from build123d import *

# Parameters (mm, degrees)
F0_R        = 30
F0_R_2      = 5
F1_DEPTH    = 4
F2_R        = 30
F3_R        = 30
F4_T1_DEPTH = 8
F5_R        = 30
F5_R_2      = 24
F6_DEPTH    = 30
F0_R_3      = 13
F7_DEPTH    = 20


# Not quite as in the source:
# - a fillet or chamfer that OpenCascade refuses, or shapes differently, is made with other operations: its cross-section is extruded or revolved along the edge and cut away or added


with BuildPart() as f1:
    # F0 (on Front) → F1 (new body, symmetric)
    with BuildSketch(Plane.XZ):
        with BuildLine():
            ThreePointArc((34.9249194702, -19.5), (38.7104428986, -10.074800772), (40, 0))
            ThreePointArc((40, 0), (38.7104428986, 10.074800772), (34.9249194702, 19.5))
            ThreePointArc((34.9249194702, 19.5), (28.892590505, 27.6625778609), (21, 34.0440890611))
            ThreePointArc((21, 34.0440890611), (0, 40), (-21, 34.0440890611))
            ThreePointArc((-21, 34.0440890611), (-27.6625778609, -28.892590505), (34.9249194702, -19.5))
        make_face()
        Circle(F0_R, mode=Mode.SUBTRACT)
        with BuildLine():
            ThreePointArc((34.9249194702, 19.5), (38.7104428986, 10.074800772), (40, 0))
            ThreePointArc((40, 0), (38.7104428986, -10.074800772), (34.9249194702, -19.5))
            Line((34.9249194702, -19.5), (206.3684774144, -12.4895628079))
            ThreePointArc((206.3684774144, -12.4895628079), (193.3577711699, 0), (206.3684774144, 12.4895628079))
            Line((206.3684774144, 12.4895628079), (34.9249194702, 19.5))
        make_face()
        with BuildLine():
            ThreePointArc((218.3577711699, 0), (214.8753603171, 8.6563898926), (206.3684774144, 12.4895628079))
            ThreePointArc((206.3684774144, 12.4895628079), (193.3577711699, 0), (206.3684774144, -12.4895628079))
            ThreePointArc((206.3684774144, -12.4895628079), (214.8753603171, -8.6563898926), (218.3577711699, 0))
        make_face()
        with Locations((205.8577711699, 0)):
            Circle(F0_R_2, mode=Mode.SUBTRACT)
        with BuildLine():
            ThreePointArc((-21, 34.0440890611), (0, 40), (21, 34.0440890611))
            Line((21, 34.0440890611), (11.5, 186.8090940417))
            ThreePointArc((11.5, 186.8090940417), (0, 182.5), (-11.5, 186.8090940417))
            Line((-11.5, 186.8090940417), (-21, 34.0440890611))
        make_face()
    extrude(amount=F1_DEPTH, both=True)

    # F2
    f2_edges = [f1.edges().sort_by_distance(p)[0] for p in [
        (-21, 0, 34.044089),
        (34.924919, 0, -19.5),
    ]]
    fillet(f2_edges, radius=F2_R)

    # F3
    f3_edges = [f1.edges().sort_by_distance(p)[0] for p in [
        (34.924919, 0, 19.5),
    ]]
    fillet(f3_edges, radius=F3_R)

    # F4: fillet of radius 30 on 1 edges, made by hand

    # F4_s2 → F4_t1 (join)
    with BuildSketch(Plane.XZ.offset(-4)):
        with BuildLine():
            ThreePointArc((28.649862751, 27.9138919599), (22.7110220839, 36.6919475661), (20.1951004828, 46.9872973509))
            Line((20.1951004828, 46.9872973509), (21, 34.0440890611))
            ThreePointArc((21, 34.0440890611), (25.0134373272, 31.2142267736), (28.649862751, 27.9138919599))
        make_face()
    extrude(amount=F4_T1_DEPTH)

    # F5 (on Front) → F6 (join, symmetric)
    with BuildSketch(Plane.XZ):
        Circle(F5_R)
        Circle(F5_R_2, mode=Mode.SUBTRACT)
    extrude(amount=F6_DEPTH, both=True)

    # F0 (on Front) → F7 (join, symmetric)
    with BuildSketch(Plane.XZ):
        with BuildLine():
            ThreePointArc((-11.5, 186.8090940417), (0, 182.5), (11.5, 186.8090940417))
            ThreePointArc((11.5, 186.8090940417), (15.9295323221, 192.7543116269), (17.5, 200))
            ThreePointArc((17.5, 200), (-7.2456883731, 215.9295323221), (-11.5, 186.8090940417))
        make_face()
        with Locations((0, 200)):
            Circle(F0_R_3, mode=Mode.SUBTRACT)
    extrude(amount=F7_DEPTH, both=True)


solid = f1.part
Input: part model. Units: mm. Frame: model coordinates. A direction names the side the tool comes from. Round coordinates to 2 decimals unless told otherwise and drop trailing zeros. Order: outer loops, then holes, each group sorted by start corner. A loop starts at its lowest first (then second) coordinate and runs counter-clockwise, first axis right, second up.
1. Cut plane B-B, the plane y = -13.5. Output: boundary loops of the cut face in (x, z).
The answers:
outline: circle Ø60 at (0, 0); circle Ø35 at (0, 200); hole circle Ø48 at (0, 0); hole circle Ø26 at (0, 200)
2. Mould query, pull axis Y, two halves, no side actions, for faces 5 (the face through (-15.787, 0.056, 117.877)), 6 (the face through (-13.5, 30, 20.1)), 7 (the face through (-3, -20, 213)). Classes: released by +Y, released by -Y, zero draft, split by the parting line, or undercut.
The answers:
face 5: zero draft
face 6: released by +Y
face 7: released by -Y
3. Cut plane C-C, the plane z = 191.5. Output: boundary loops of the cut face in (x, y).
The answers:
outline: (-15.3, -20) - (-9.84, -20) - (-9.84, 20) - (-15.3, 20) - close; (9.84, -20) - (15.3, -20) - (15.3, 20) - (9.84, 20) - close
4. Set-up query: faces 1 (the face through (-29.97, -17.18, 1.32)), 2 (the face through (-29.97, 16.82, 1.32)), 3 (the face through (15.91, -0.06, 115.92)), 4 (the face through (-23.977, 0.42, 1.055)). Return all of +Z, -Z, +X, -X, +Y, -Y with unobstructed straight access to the full face (end or side cutting, diameter ignored); none if empty.
The answers:
face 1: -Y
face 2: +Y
face 3: +X, +Y, -Y
face 4: +Y, -Y
5. Cut plane A-A, the plane x = 0. Output: boundary loops of the cut face in (y, z), then the cut area to 3 significant figures.
The answers:
outline: (-30, -30) - (-4, -30) - (-4, -40) - (4, -40) - (4, -30) - (30, -30) - (30, -24) - (-30, -24) - close; (-30, 24) - (30, 24) - (30, 30) - (4, 30) - (4, 182.5) - (20, 182.5) - (20, 187) - (-20, 187) - (-20, 182.5) - (-4, 182.5) - (-4, 30) - (-30, 30) - close; (-20, 213) - (20, 213) - (20, 217.5) - (-20, 217.5) - close
area: 2,380 mm2
6. Pin query (flat end, axial travel): P1, Ø12, axis at y = -20.5, z = 181, coming from the +X side; P2, Ø6, axis at x = 118.5, y = -5.5, coming from the -Z side; P3, Ø13, axis at x = 205.86, z = 0, coming from the -Y side; P4, Ø1, axis at y = 6, z = 165.5, coming from the -X side (1 decimal). Return the tip coordinate at first contact, or that it passes through.
The answers:
P1: stops at x = 11.69
P2: stops at z = -16.19
P3: stops at y = -4
P4: passes through
7. Material intervals for line 1 (Z direction, x = 0, y = 13); line 2 (Z direction, x = 0, y = -2.5); line 3 (Z direction, x = -18, y = 12.5), sorted ascending.
The answers:
line 1: z = -30 to -24, 24 to 30, 182.5 to 187, 213 to 217.5
line 2: z = -40 to -24, 24 to 187, 213 to 217.5
line 3: z = -24 to -15.87, 15.87 to 24
8. Cut plane D-D, the plane z = 55.5. Output: boundary loops of the cut face in (x, y), then the cut area to 3 significant figures.
The answers:
outline: (-19.67, -4) - (19.67, -4) - (19.67, 4) - (-19.67, 4) - close
area: 315 mm2
